```python
from build123d import *

# Parameters (mm, degrees)
F0_R        = 1.5
F0_R_2      = 3.5
F1_DEPTH    = 1.5
F2_T1_DEPTH = 1.5
F2_T3_DEPTH = 6.6314425489
F2_T5_DEPTH = 7.4016994375
F2_T7_DEPTH = 2.253003807
F4_DEPTH    = 25
F5_R        = 2
F6_R        = 3


# Not quite as in the source:
# - a fillet or chamfer that OpenCascade refuses, or shapes differently, is made with other operations: its cross-section is extruded or revolved along the edge and cut away or added


with BuildPart() as f1:
    # F0 (on Top) → F1 (new body)
    with BuildSketch(Plane.XY):
        with BuildLine():
            Line((-17, 42), (-20, 36))
            Line((-20, 36), (-20, -36))
            Line((-20, -36), (-17, -42))
            Line((-17, -42), (-17, -45.25))
            Line((-17, -45.25), (-14, -52.25))
            Line((-14, -52.25), (-9, -52.25))
            Line((-9, -52.25), (-7.9737930839, -39.6029885204))
            ThreePointArc((-7.9737930839, -39.6029885204), (0, -32.25), (7.9737930839, -39.6029885204))
            Line((7.9737930839, -39.6029885204), (9, -52.25))
            Line((9, -52.25), (14, -52.25))
            Line((14, -52.25), (17, -45.25))
            Line((17, -45.25), (17, -42))
            Line((17, -42), (20, -36))
            Line((20, -36), (20, 36))
            Line((20, 36), (17, 42))
            Line((17, 42), (17, 45.25))
            Line((17, 45.25), (14, 52.25))
            Line((14, 52.25), (4.468852459, 71.2426229508))
            ThreePointArc((4.468852459, 71.2426229508), (0, 74), (-4.468852459, 71.2426229508))
            Line((-4.468852459, 71.2426229508), (-14, 52.25))
            Line((-14, 52.25), (-17, 45.25))
            Line((-17, 45.25), (-17, 42))
        make_face()
        with Locations((-12.5, -45.25)):
            Circle(F0_R, mode=Mode.SUBTRACT)
        with Locations((-15.25, -15.25)):
            Circle(F0_R, mode=Mode.SUBTRACT)
        with Locations((12.5, -45.25)):
            Circle(F0_R, mode=Mode.SUBTRACT)
        with Locations((15.25, -15.25)):
            Circle(F0_R, mode=Mode.SUBTRACT)
        with Locations((-15.25, 15.25)):
            Circle(F0_R, mode=Mode.SUBTRACT)
        with BuildLine():
            Line((-16, 28), (-16, 31))
            ThreePointArc((-16, 31), (-15, 32), (-14, 31))
            Line((-14, 31), (-14, 28))
            ThreePointArc((-14, 28), (-15, 27), (-16, 28))
        make_face(mode=Mode.SUBTRACT)
        with BuildLine():
            Line((-6.5694088498, 53.6796721311), (-8.1392449154, 50.5514754098))
            ThreePointArc((-8.1392449154, 50.5514754098), (-9.4815399974, 50.1062295082), (-9.926785899, 51.4485245902))
            Line((-9.926785899, 51.4485245902), (-8.3569498334, 54.5767213115))
            ThreePointArc((-8.3569498334, 54.5767213115), (-7.0146547515, 55.0219672131), (-6.5694088498, 53.6796721311))
        make_face(mode=Mode.SUBTRACT)
        with Locations((15.25, 15.25)):
            Circle(F0_R, mode=Mode.SUBTRACT)
        with BuildLine():
            ThreePointArc((16, 28), (15, 27), (14, 28))
            Line((14, 28), (14, 31))
            ThreePointArc((14, 31), (15, 32), (16, 31))
            Line((16, 31), (16, 28))
        make_face(mode=Mode.SUBTRACT)
        with BuildLine():
            ThreePointArc((9.926785899, 51.4485245902), (9.4815399974, 50.1062295082), (8.1392449154, 50.5514754098))
            Line((8.1392449154, 50.5514754098), (6.5694088498, 53.6796721311))
            ThreePointArc((6.5694088498, 53.6796721311), (7.0146547515, 55.0219672131), (8.3569498334, 54.5767213115))
            Line((8.3569498334, 54.5767213115), (9.926785899, 51.4485245902))
        make_face(mode=Mode.SUBTRACT)
        with Locations((0, 60)):
            Circle(F0_R_2, mode=Mode.SUBTRACT)
        with Locations((0, 69)):
            Circle(F0_R, mode=Mode.SUBTRACT)
    extrude(amount=F1_DEPTH)

    # F2: fillet of radius 5 on 14 edges, made by hand

    # F2_s2 → F2_t1 (join)
    with BuildSketch(Plane.XY):
        with BuildLine():
            ThreePointArc((-17, 43.1803398875), (-17.1337550527, 42.0315752848), (-17.527864045, 40.94427191))
            Line((-17.527864045, 40.94427191), (-17, 42))
            Line((-17, 42), (-17, 43.1803398875))
        make_face()
        with BuildLine():
            ThreePointArc((17.527864045, 40.94427191), (17.1337550527, 42.0315752848), (17, 43.1803398875))
            Line((17, 43.1803398875), (17, 42))
            Line((17, 42), (17.527864045, 40.94427191))
        make_face()
        with BuildLine():
            ThreePointArc((17, -43.1803398875), (17.1337550527, -42.0315752848), (17.527864045, -40.94427191))
            Line((17.527864045, -40.94427191), (17, -42))
            Line((17, -42), (17, -43.1803398875))
        make_face()
        with BuildLine():
            ThreePointArc((-17.527864045, -40.94427191), (-17.1337550527, -42.0315752848), (-17, -43.1803398875))
            Line((-17, -43.1803398875), (-17, -42))
            Line((-17, -42), (-17.527864045, -40.94427191))
        make_face()
    extrude(amount=F2_T1_DEPTH)

    # F2_s4 → F2_t3 (cut)
    with BuildSketch(Plane.XY.offset(-2.5657212744)):
        with BuildLine():
            ThreePointArc((16.5957251501, -46.1933079831), (16.897888614, -45.2290408516), (17, -44.2237114902))
            Line((17, -44.2237114902), (17, -45.25))
            Line((17, -45.25), (16.5957251501, -46.1933079831))
        make_face()
        with BuildLine():
            ThreePointArc((-16.5957251501, 46.1933079831), (-16.897888614, 45.2290408516), (-17, 44.2237114902))
            Line((-17, 44.2237114902), (-17, 45.25))
            Line((-17, 45.25), (-16.5957251501, 46.1933079831))
        make_face()
        with BuildLine():
            ThreePointArc((16.5957251501, 46.1933079831), (16.897888614, 45.2290408516), (17, 44.2237114902))
            Line((17, 44.2237114902), (17, 45.25))
            Line((17, 45.25), (16.5957251501, 46.1933079831))
        make_face()
        with BuildLine():
            ThreePointArc((-17, -44.2237114902), (-16.897888614, -45.2290408516), (-16.5957251501, -46.1933079831))
            Line((-16.5957251501, -46.1933079831), (-17, -45.25))
            Line((-17, -45.25), (-17, -44.2237114902))
        make_face()
    extrude(amount=F2_T3_DEPTH, mode=Mode.SUBTRACT)

    # F2_s6 → F2_t5 (cut)
    with BuildSketch(Plane.XY.offset(-2.9508497187)):
        with BuildLine():
            ThreePointArc((-19.472135955, 37.05572809), (-19.8662449473, 35.9684247152), (-20, 34.8196601125))
            Line((-20, 34.8196601125), (-20, 36))
            Line((-20, 36), (-19.472135955, 37.05572809))
        make_face()
        with BuildLine():
            ThreePointArc((20, 34.8196601125), (19.8662449473, 35.9684247152), (19.472135955, 37.05572809))
            Line((19.472135955, 37.05572809), (20, 36))
            Line((20, 36), (20, 34.8196601125))
        make_face()
        with BuildLine():
            ThreePointArc((19.472135955, -37.05572809), (19.8662449473, -35.9684247152), (20, -34.8196601125))
            Line((20, -34.8196601125), (20, -36))
            Line((20, -36), (19.472135955, -37.05572809))
        make_face()
        with BuildLine():
            ThreePointArc((-20, -34.8196601125), (-19.8662449473, -35.9684247152), (-19.472135955, -37.05572809))
            Line((-19.472135955, -37.05572809), (-20, -36))
            Line((-20, -36), (-20, -34.8196601125))
        make_face()
    extrude(amount=F2_T5_DEPTH, mode=Mode.SUBTRACT)

    # F2_s8 → F2_t7 (cut)
    with BuildSketch(Plane.XY.offset(-0.3765019035)):
        with BuildLine():
            ThreePointArc((-13.9324518552, 52.3846025166), (-13.9979436343, 52.2490444272), (-14.0593245463, 52.1115760587))
            Line((-14.0593245463, 52.1115760587), (-14, 52.25))
            Line((-14, 52.25), (-13.9324518552, 52.3846025166))
        make_face()
        with BuildLine():
            ThreePointArc((13.9324518552, 52.3846025166), (13.9979436343, 52.2490444272), (14.0593245463, 52.1115760587))
            Line((14.0593245463, 52.1115760587), (14, 52.25))
            Line((14, 52.25), (13.9324518552, 52.3846025166))
        make_face()
    extrude(amount=F2_T7_DEPTH, mode=Mode.SUBTRACT)

    # F3 (on face) → F4 (cut)
    with BuildSketch(Plane.XY.offset(1.5)):
        with BuildLine():
            Line((-14, -27.25), (-15, -27.25))
            ThreePointArc((-15, -27.25), (-15.5, -27.75), (-15, -28.25))
            Line((-15, -28.25), (-15, -34.25))
            ThreePointArc((-15, -34.25), (-15.5, -34.75), (-15, -35.25))
            Line((-15, -35.25), (-14, -35.25))
            ThreePointArc((-14, -35.25), (-13.5, -34.75), (-14, -34.25))
            Line((-14, -34.25), (-14, -28.25))
            ThreePointArc((-14, -28.25), (-13.5, -27.75), (-14, -27.25))
        make_face()
        with BuildLine():
            Line((14, -35.25), (15, -35.25))
            ThreePointArc((15, -35.25), (15.5, -34.75), (15, -34.25))
            Line((15, -34.25), (15, -28.25))
            ThreePointArc((15, -28.25), (15.5, -27.75), (15, -27.25))
            Line((15, -27.25), (14, -27.25))
            ThreePointArc((14, -27.25), (13.5, -27.75), (14, -28.25))
            Line((14, -28.25), (14, -34.25))
            ThreePointArc((14, -34.25), (13.5, -34.75), (14, -35.25))
        make_face()
    extrude(amount=-F4_DEPTH, mode=Mode.SUBTRACT)

    # F5
    f5_edges = [f1.edges().sort_by_distance(p)[0] for p in [
        (-9, -52.25, 0.75),
        (9, -52.25, 0.75),
    ]]
    fillet(f5_edges, radius=F5_R)

    # F6
    f6_edges = [f1.edges().sort_by_distance(p)[0] for p in [
        (-14, -52.25, 0.75),
        (14, -52.25, 0.75),
    ]]
    fillet(f6_edges, radius=F6_R)


solid = f1.part
```
Source: CAD feature listing. Evaluate the final solid. Frame: model axes, mm. Give positions to 0.01 mm unless a question says otherwise; leave off trailing zeros. Order: outer loops, then holes, each group sorted by start corner. A loop starts at its lowest first (then second) coordinate and runs counter-clockwise, first axis right, second up.
(1) Material intervals for line 1 along X through (y, z) = (-15.5, 0.45); line 2 along X through (y, z) = (-34, 0.1); line 3 along Y through (x, z) = (12.5, 0.9), sorted ascending.
(2) Contact query for flat-ended pins moving along their axis: P1, Ø0.5, axis at x = -14.5, z = 1, coming from the +Y side; P2, Ø2.5, axis at x = -15.25, y = 15.25, coming from the -Z side. Output: stop coordinate, or through.
(3) Section query C-C (z = 0.4). State how many separate pieces and enclosed holes the cut face has, plus the area to 3 significant figures.
(4) Pull-direction query (X, two-part tool) for faces 1 (the face through (13.75, 15.32, 0.74)), 2 (the face through (0, 12, 1.5)), 3 (the face through (15.345, 49.111, 0.74)), 4 (the face through (-9.13, 61.95, 0.74)); classes: +X half, -X half, draft (parallel to the pull), parting line (faces both ways), or undercut.
(5) Section query B-B (x = 0). Return the cut outline in (y, z).
(6) Section query D-D (y = 65.5). Return the cut outline in (x, z), plus the area to 3 significant figures.
(7) Section query A-A (y = 15.25). Return the cut outline in (x, z).
Outcome:
1. line 1: x = -20 to -16.73, -13.77 to 13.77, 16.73 to 20
1. line 2: x = -20 to -15, -14 to -4.99, 4.99 to 14, 15 to 20
1. line 3: y = -52.21 to -46.75, -43.75 to 55.24
2. P1: stops at y = 51.67
2. P2: passes through
3. separate pieces: 1
3. enclosed holes: 14
3. area: 3,890 mm2
4. face 1: undercut
4. face 2: draft
4. face 3: +X half
4. face 4: -X half
5. outline: (-32.25, 0) - (56.5, 0) - (56.5, 1.5) - (-32.25, 1.5) - close; (63.5, 0) - (67.5, 0) - (67.5, 1.5) - (63.5, 1.5) - close; (70.5, 0) - (74, 0) - (74, 1.5) - (70.5, 1.5) - close
6. outline: (-7.35, 0) - (7.35, 0) - (7.35, 1.5) - (-7.35, 1.5) - close
6. area: 22.1 mm2
7. outline: (-20, 0) - (-16.75, 0) - (-16.75, 1.5) - (-20, 1.5) - close; (-13.75, 0) - (13.75, 0) - (13.75, 1.5) - (-13.75, 1.5) - close; (16.75, 0) - (20, 0) - (20, 1.5) - (16.75, 1.5) - close
